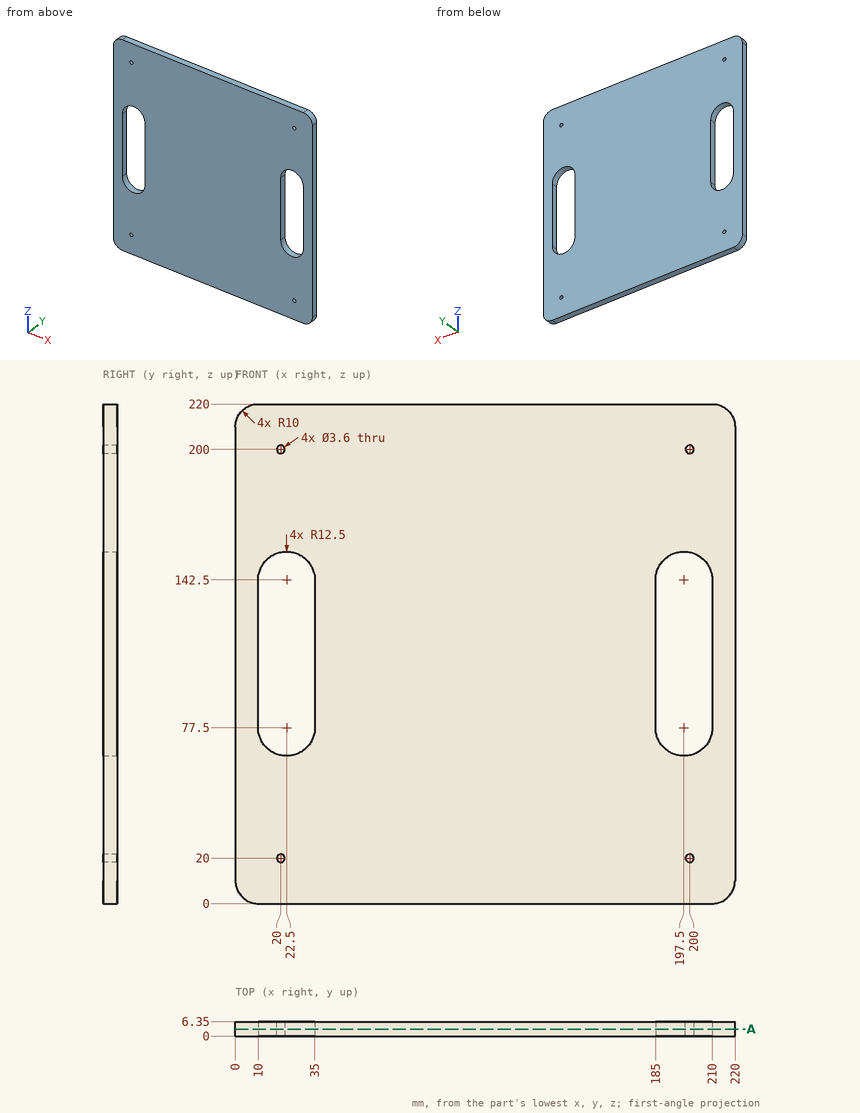
Check sheet for the drawn part. Datum: minimum x, y, z corner. Units: mm. Give positions to 0.01 mm unless a question says otherwise; leave off trailing zeros. Loops run counter-clockwise (first coordinate to the right, second up) from the corner with the lowest first, then second, coordinate; pieces in that order, holes last.
1) Thickness scan on line 1 along X through (y, z) = (3.25, 120); line 2 along X through (y, z) = (2.5, 200); line 3 along Z through (x, y) = (200, 1.5). Record the ranges inside material, lowest first.
2) Depth check by flat-ended pin: pin 1 Ø4.5 at (x, z) = (200, 20) entering from -Y. Enter the tip coordinate at first touch or a pass-through.
3) Sectioned sample at A-A, the plane y = 3. Enter the section's corners in (x, z), then the cut area to 3 significant figures.
Answers:
1. line 1: x = 0 to 10, 35 to 185, 210 to 220
1. line 2: x = 0 to 18.2, 21.8 to 198.2, 201.8 to 220
1. line 3: z = 0 to 18.2, 21.8 to 65.25, 154.75 to 198.2, 201.8 to 220
2. pin 1: stops at y = 0
3. outline: (0, 10) arc R10 ccw to (10, 0) - (210, 0) arc R10 ccw to (220, 10) - (220, 210) arc R10 ccw to (210, 220) - (10, 220) arc R10 ccw to (0, 210) - close; hole (10, 77.5) arc R12.5 ccw to (35, 77.5) - (35, 142.5) arc R12.5 ccw to (10, 142.5) - close; hole circle Ø3.6 at (20, 20); hole circle Ø3.6 at (20, 200); hole (185, 77.5) arc R12.5 ccw to (210, 77.5) - (210, 142.5) arc R12.5 ccw to (185, 142.5) - close; hole circle Ø3.6 at (200, 20); hole circle Ø3.6 at (200, 200)
3. area: 44,000 mm2
